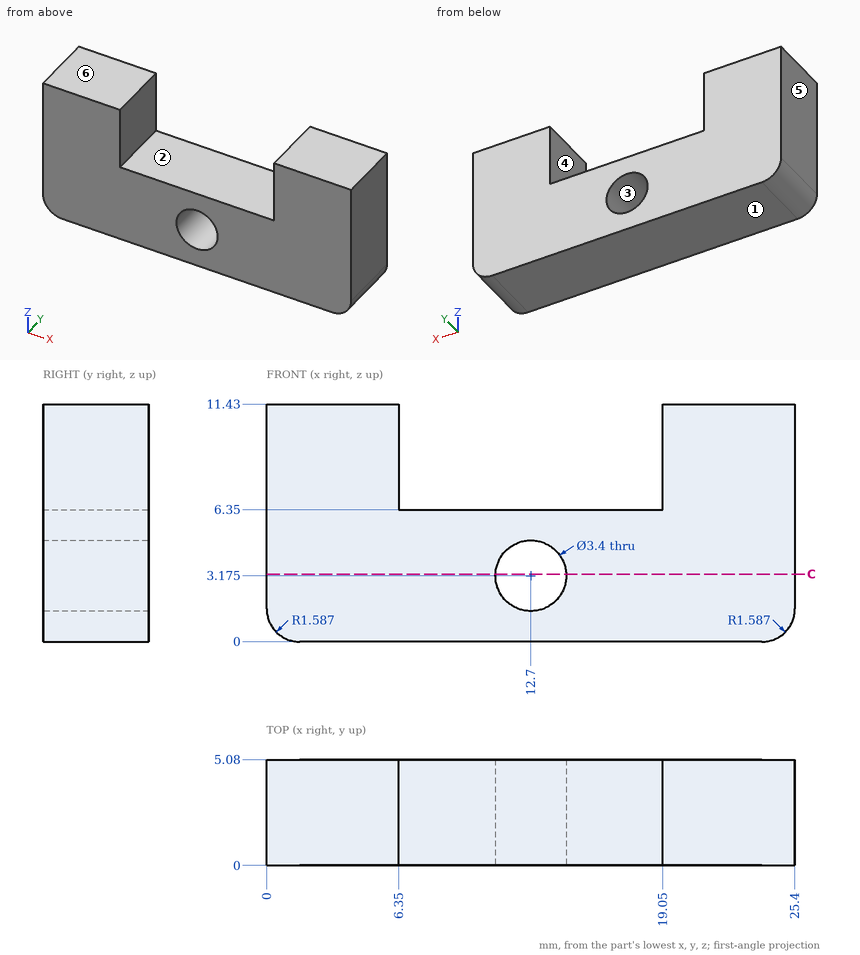
Part print with two shaded views. Sizes in mm from the minimum x, y, z corner. A direction names the side the tool comes from. Round coordinates to 2 decimals unless told otherwise and drop trailing zeros. Loops run counter-clockwise (first coordinate to the right, second up) from the corner with the lowest first, then second, coordinate; pieces in that order, holes last.
1. Flat gauge pins, fed straight in: pin 1 (2.5 mm diameter, centred on x = 13, y = 2, fed in from +Z); pin 2 (2 mm diameter, centred on x = 8, z = 8.5, fed in from +Y). Where does each tip first touch, or does it go through?
Solutions:
pin 1: stops at z = 6.35
pin 2: passes through
2. Drill centre lines: line 1 along X through (y, z) = (1.55, 6.75); line 2 along X through (y, z) = (2.55, 3); line 3 along Z through (x, y) = (11.5, 1.25). Where is each one in solid material? Low to high.
Solutions:
line 1: x = 0 to 6.35, 19.05 to 25.4
line 2: x = 0 to 11.01, 14.39 to 25.4
line 3: z = 0 to 1.97, 4.38 to 6.35
3. Slice it at C-C (z = 3.25). Give the cut face in (x, y).
Solutions:
outline: (0, 0) - (11, 0) - (11, 5.08) - (0, 5.08) - close; (14.4, 0) - (25.4, 0) - (25.4, 5.08) - (14.4, 5.08) - close
4. 3-axis set-ups, long thin cutter, end or side, ignore diameter. For the marked faces 1 and 2: which of +Z, -Z, +X, -X, +Y, -Y reach the whole face in a straight line?
Solutions:
face 1: -Z, +X, -X, +Y, -Y
face 2: +Z, +Y, -Y
5. Two-plate mould, pull along X, no slides. Class the marked faces 3, 4, 5 and 6: pulls with the +X half, pulls with the -X half, needs draft (parallel to the pull), parting line crosses it, or undercut.
Solutions:
face 3: undercut
face 4: undercut
face 5: pulls with the -X half
face 6: needs draft
